For this review, use the dimensioned drawing (mm, ordinates from the lowest corner) and the shaded views. A direction names the side the tool comes from. Coordinates: 2 decimals unless noted, no trailing zeros. Write each loop counter-clockwise with the first axis right and the second up, starting at its lowest first coordinate (ties: lowest second). Pieces come first, ordered by that corner, then holes. Notation, with made-up numbers: M -28.75,49 L -11.75,49 A11 ccw -11.75,55 Z; hole C 57.5,88 d1. An arc over 180 degrees is marked long. One line per question, with ' | ' between items.
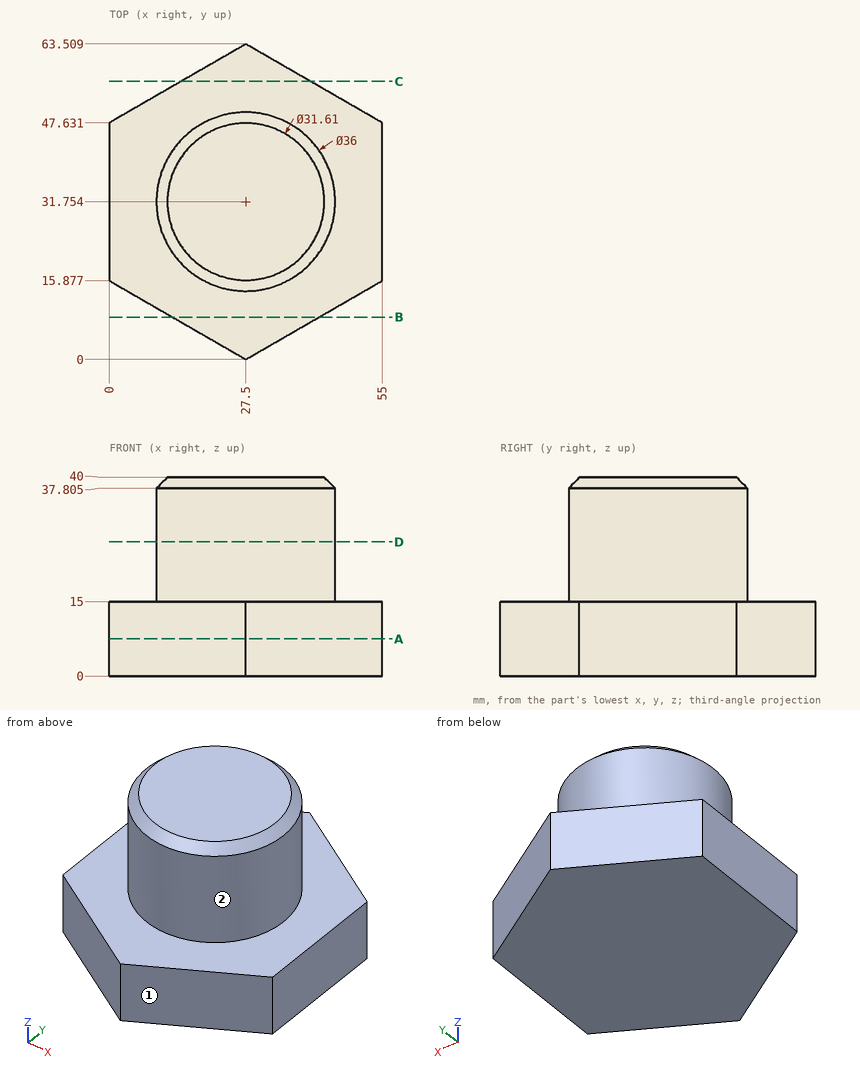
1. Take a section at B-B (y = 8.5). Write out the cut boundary in (x, z), then the cut area to 3 significant figures.
Answer sheet:
outline: M 12.78,0 L 42.22,0 L 42.22,15 L 12.78,15 Z | area: 442 mm^2
2. Tool access review of the marked faces 1 and 2: name each direction out of +Z, -Z, +X, -X, +Y, -Y from which nothing blocks a thin tool from reaching the whole face with its end or side.
Answer sheet:
face 1: +Z, -Z, +X, -Y | face 2: +Z
3. Take a section at A-A (z = 7.5). Write out the cut boundary in (x, y), then the cut area to 3 significant figures.
Answer sheet:
outline: M 0,15.88 L 27.5,0 L 55,15.88 L 55,47.63 L 27.5,63.51 L 0,47.63 Z | area: 2,620 mm^2
4. Take a section at C-C (y = 56). Write out the cut boundary in (x, z) (1 decimal).
Answer sheet:
outline: M 14.5,0 L 40.5,0 L 40.5,15 L 14.5,15 Z
5. To check wall thickness, follow line 1 along Z through (x, y) = (25, 59); line 2 along Y through (x, z) = (15, 14.5) (1 decimal); line 3 along Y through (x, z) = (38.5, 32) (1 decimal). State the ranges of each line that lie inside material, in increasing order. Write a range as [from, to].
Answer sheet:
line 1: [0, 15] | line 2: [7.2, 56.3] | line 3: [17.5, 46]
6. Take a section at D-D (z = 27). Write out the cut boundary in (x, y) (1 decimal).
Answer sheet:
outline: C 27.5,31.8 d36
7. Insertion check: pin 1 Ø4 at (x, z) = (28, 22) entering from -Y; pin 2 Ø3 at (x, y) = (12, 13.5) entering from +Z; pin 3 Ø2 at (x, z) = (38, 6) entering from +Y (1 decimal); pin 4 Ø1.5 at (x, y) = (43, 8) entering from +Z. Each pin has a flat end and moves straight along its axis. Give the tip position at first contact, or say it passes through.
Answer sheet:
pin 1: y = 13.75 | pin 2: z = 15 | pin 3: y = 58 | pin 4: through
